```python
from build123d import *

# Parameters (mm, degrees)
SKETCH1_R           = 3
SKETCH1_R_2         = 34
BOSS_EXTRUDE1_DEPTH = 5
BOSS_EXTRUDE2_START = 5
SKETCH2_R           = 60
SKETCH2_R_2         = 10
BOSS_EXTRUDE2_DEPTH = 5
SKETCH3_R           = 2
CUT_EXTRUDE1_DEPTH  = 35
SKETCH5_R           = 35.5
CUT_EXTRUDE3_DEPTH  = 5
SKETCH6_R           = 35.5
CUT_EXTRUDE4_DEPTH  = 3
SKETCH7_R           = 93.527900111
SKETCH7_R_2         = 60
CUT_EXTRUDE5_DEPTH  = 10


with BuildPart() as part:
    # Sketch1 → Boss-Extrude1 (new body)
    with BuildSketch(Plane.XY):
        with BuildLine():
            ThreePointArc((59.930310696, 2.890996349), (-60, 0), (59.930310696, -2.890996349))
            ThreePointArc((59.930310696, -2.890996349), (62.891836179, 0), (59.930310696, 2.890996349))
        make_face()
        with Locations((44, 0)):
            Circle(SKETCH1_R, mode=Mode.SUBTRACT)
        with Locations((43.099317415, -8.857134884)):
            Circle(SKETCH1_R, mode=Mode.SUBTRACT)
        with Locations((40.434143711, -17.351657625)):
            Circle(SKETCH1_R, mode=Mode.SUBTRACT)
        with Locations((36.113591413, -25.135801464)):
            Circle(SKETCH1_R, mode=Mode.SUBTRACT)
        with Locations((30.314544439, -31.890882638)):
            Circle(SKETCH1_R, mode=Mode.SUBTRACT)
        with Locations((23.274416454, -37.34034733)):
            Circle(SKETCH1_R, mode=Mode.SUBTRACT)
        with Locations((15.281431125, -41.261093814)):
            Circle(SKETCH1_R, mode=Mode.SUBTRACT)
        with Locations((6.66282221, -43.49260627)):
            Circle(SKETCH1_R, mode=Mode.SUBTRACT)
        with Locations((-2.228563429, -43.943526316)):
            Circle(SKETCH1_R, mode=Mode.SUBTRACT)
        with Locations((-11.028711419, -42.59539323)):
            Circle(SKETCH1_R, mode=Mode.SUBTRACT)
        with Locations((-19.377342669, -39.503399741)):
            Circle(SKETCH1_R, mode=Mode.SUBTRACT)
        with Locations((-26.932663232, -34.794132425)):
            Circle(SKETCH1_R, mode=Mode.SUBTRACT)
        with Locations((-33.385357398, -28.66038924)):
            Circle(SKETCH1_R, mode=Mode.SUBTRACT)
        with Locations((-38.47125111, -21.353286351)):
            Circle(SKETCH1_R, mode=Mode.SUBTRACT)
        with Locations((-41.982127282, -13.171977411)):
            Circle(SKETCH1_R, mode=Mode.SUBTRACT)
        with Locations((-43.774250229, -4.451406167)):
            Circle(SKETCH1_R, mode=Mode.SUBTRACT)
        with Locations((-43.774250229, 4.451406167)):
            Circle(SKETCH1_R, mode=Mode.SUBTRACT)
        with Locations((-41.982127282, 13.171977411)):
            Circle(SKETCH1_R, mode=Mode.SUBTRACT)
        with Locations((-38.47125111, 21.353286351)):
            Circle(SKETCH1_R, mode=Mode.SUBTRACT)
        with Locations((-33.385357398, 28.66038924)):
            Circle(SKETCH1_R, mode=Mode.SUBTRACT)
        with Locations((-26.932663232, 34.794132425)):
            Circle(SKETCH1_R, mode=Mode.SUBTRACT)
        with Locations((-19.377342669, 39.503399741)):
            Circle(SKETCH1_R, mode=Mode.SUBTRACT)
        with Locations((-11.028711419, 42.59539323)):
            Circle(SKETCH1_R, mode=Mode.SUBTRACT)
        with Locations((-2.228563429, 43.943526316)):
            Circle(SKETCH1_R, mode=Mode.SUBTRACT)
        with Locations((6.66282221, 43.49260627)):
            Circle(SKETCH1_R, mode=Mode.SUBTRACT)
        with Locations((15.281431125, 41.261093814)):
            Circle(SKETCH1_R, mode=Mode.SUBTRACT)
        with Locations((23.274416454, 37.34034733)):
            Circle(SKETCH1_R, mode=Mode.SUBTRACT)
        with Locations((30.314544439, 31.890882638)):
            Circle(SKETCH1_R, mode=Mode.SUBTRACT)
        with Locations((36.113591413, 25.135801464)):
            Circle(SKETCH1_R, mode=Mode.SUBTRACT)
        with Locations((40.434143711, 17.351657625)):
            Circle(SKETCH1_R, mode=Mode.SUBTRACT)
        with Locations((43.099317415, 8.857134884)):
            Circle(SKETCH1_R, mode=Mode.SUBTRACT)
        Circle(SKETCH1_R_2, mode=Mode.SUBTRACT)
    extrude(amount=BOSS_EXTRUDE1_DEPTH)

    # Sketch2 → Boss-Extrude2 (add)
    with BuildSketch(Plane(origin=(0, 0, 0), x_dir=(-1, 0, 0), z_dir=(0, 0, -1)).offset(BOSS_EXTRUDE2_START)):
        Circle(SKETCH2_R)
        Circle(SKETCH2_R_2, mode=Mode.SUBTRACT)
    extrude(amount=-BOSS_EXTRUDE2_DEPTH)

    # Sketch3 → Cut-Extrude1 (cut)
    with BuildSketch(Plane.XY.offset(5)):
        with Locations((0, 54)):
            Circle(SKETCH3_R)
        with Locations((38.183766184, 38.183766184)):
            Circle(SKETCH3_R)
        with Locations((54, 0)):
            Circle(SKETCH3_R)
        with Locations((38.183766184, -38.183766184)):
            Circle(SKETCH3_R)
        with Locations((0, -54)):
            Circle(SKETCH3_R)
        with Locations((-38.183766184, -38.183766184)):
            Circle(SKETCH3_R)
        with Locations((-54, 0)):
            Circle(SKETCH3_R)
        with Locations((-38.183766184, 38.183766184)):
            Circle(SKETCH3_R)
    extrude(amount=-CUT_EXTRUDE1_DEPTH, mode=Mode.SUBTRACT)

    # Sketch5 → Cut-Extrude3 (cut)
    with BuildSketch(Plane(origin=(0, 0, -5), x_dir=(-1, 0, 0), z_dir=(0, 0, -1))):
        Circle(SKETCH5_R)
    extrude(amount=-CUT_EXTRUDE3_DEPTH, mode=Mode.SUBTRACT)

    # Sketch6 → Cut-Extrude4 (cut)
    with BuildSketch(Plane(origin=(0, 0, 0), x_dir=(-1, 0, 0), z_dir=(0, 0, -1))):
        Circle(SKETCH6_R)
    extrude(amount=-CUT_EXTRUDE4_DEPTH, mode=Mode.SUBTRACT)

    # Sketch7 → Cut-Extrude5 (cut)
    with BuildSketch(Plane(origin=(0, 0, -5), x_dir=(-1, 0, 0), z_dir=(0, 0, -1))):
        Circle(SKETCH7_R)
        Circle(SKETCH7_R_2, mode=Mode.SUBTRACT)
    extrude(amount=-CUT_EXTRUDE5_DEPTH, mode=Mode.SUBTRACT)


solid = part.part
```
Check sheet for the modelled part. Datum: model origin and axes. Units: mm. A direction names the side the tool comes from. Coordinates: 2 decimals unless noted, no trailing zeros. Write each loop counter-clockwise with the first axis right and the second up, starting at its lowest first coordinate (ties: lowest second). Pieces come first, ordered by that corner, then holes. Notation, with made-up numbers: M 41,28.5 L 97,28.5 A23 ccw 97,67.5 Z; hole C 45.5,-25.5 d7. An arc over 180 degrees is marked long. Write item = value, one per line. Start each with the question number.
1. Mould release check, pull along Y, two halves, no side actions. Record for faces 1 (the cylindrical face through (-41.47, -21.22, 2.46)), 2 (the cylindrical face through (-35.596, 30.688, 2.465)): pulls with the +Y half, pulls with the -Y half, needs draft (parallel to the pull), parting line crosses it, or undercut.
2. Go/stop test with flat-tipped pins: pin 1 (12 mm diameter, centred on x = -19.5, y = -18.5, fed in from -Z); pin 2 (3 mm diameter, centred on x = 23.5, y = -37, fed in from +Z); pin 3 (2 mm diameter, centred on y = -43, z = -1.5, fed in from -X); pin 4 (6 mm diameter, centred on y = 47.5, z = 3.5, fed in from +X). Record where each tip stops, or that it passes through.
3. Sectioned sample at B-B (z = -2). State how many separate pieces and enclosed holes the cut face has, then the cut area to 3 significant figures.
4. Sectioned sample at C-C (y = 0). Record the cut outline in (x, z).
5. Tool access check on faces 3 (the cylindrical face through (37.75, -40.136, 0.07)), 4 (the flat face through (-42, 13, 0)). Record the directions out of +Z, -Z, +X, -X, +Y, -Y that give a thin tool (end or side, any length) a straight path to the whole face; none if there is none.
6. Thickness scan on probe 1 along X at (y, z) = (9, 0.25); probe 2 along X at (y, z) = (-9, 3.75); probe 3 along Y at (x, z) = (13, 2.25). Record the ranges inside material, lowest first.
7. Sectioned sample at A-A (y = -54). Record the cut outline in (x, z).
The answers:
q1.face_1 = undercut
q1.face_2 = undercut
q2.pin_1 = through
q2.pin_2 = 0
q2.pin_3 = -42.85
q2.pin_4 = 40.25
q3.separate_pieces = 1
q3.enclosed_holes = 9
q3.area = 7,250 mm²
q4.outline = M -60,-5 L -56,-5 L -56,5 L -60,5 Z; M -52,-5 L -35.5,-5 L -35.5,3 L -34,3 L -34,5 L -52,5 Z; M 34,3 L 35.5,3 L 35.5,-5 L 52,-5 L 52,5 L 47,5 L 47,0 L 41,0 L 41,5 L 34,5 Z; M 56,-5 L 60,-5 L 60,5 L 56,5 Z
q5.face_3 = +Z, -Z
q5.face_4 = +Z
q6.probe_1 = -59.32 to -34.34, 34.34 to 40.1, 46.1 to 59.32
q6.probe_2 = -59.32 to -32.79, 32.79 to 40.1, 46.1 to 59.32
q6.probe_3 = -58.57 to -43.21, -39.31 to -33.03, 33.03 to 39.31, 43.21 to 58.57
q7.outline = M -26.15,-5 L -2,-5 L -2,5 L -26.15,5 Z; M 2,-5 L 26.15,-5 L 26.15,5 L 2,5 Z
